Geometry check sheet. Reference: the model listing, model coordinates, mm. Round coordinates to 2 decimals unless told otherwise and drop trailing zeros. Order: outer loops, then holes, each group sorted by start corner. A loop starts at its lowest first (then second) coordinate and runs counter-clockwise, first axis right, second up. Notation, with made-up numbers: M 10.5,80 L 26.5,80 A17 ccw 26.5,100 Z; hole C 53,-10 d5. An arc over 180 degrees is marked long. Return JSON: item names as keys, results as strings. Group by question number.
Autodesk Inventor part; units mm, degrees
ref_plane "YZ Plane" through (0, 0, 0) normal (1, 0, 0) x (0, 1, 0)
ref_plane "XZ Plane" through (0, 0, 0) normal (0, 1, 0) x (-1, 0, 0)
ref_plane "XY Plane" through (0, 0, 0) normal (0, 0, 1) x (1, 0, 0)
sketch "Sketch1" plane through (0, 0, 0) normal (0, 1, 0) x (-1, 0, 0)
  line L0 (0, 0) -> (127, 0)
  line L1 (127, 0) -> (127, -152.4)
  line L2 (127, -152.4) -> (0, -152.4)
  line L3 (0, -152.4) -> (0, 0)
  line L4 (127, -65.405) -> (25.4, -65.405)
  line L5 (25.4, -65.405) -> (25.4, -86.995)
  line L6 (25.4, -86.995) -> (127, -86.995)
  line L7 (127, -86.995) -> (127, -65.405)
  dimension "d0" = 152.4
  dimension "d1" = 127
  dimension "d2" = 21.59
  dimension "d3" = 65.405
  dimension "d4" = 101.6
extrude "Extrusion1" add sketch "Sketch1" along normal blind 1.8542 contours L0 L1 L4 L5 L6 L2 L3
equation "\"d3\" = -0.5 * d2 + 0.5 * d0"
properties part number "paddle collection ramp"
Q1. Section check B-B on y = 1.1. Record the cut outline in (x, z) (3 decimals), plus the area to 3 significant figures.
Q2. Material ranges on line 1 along Z through (x, y) = (-106, 0.4) (3 decimals); line 2 along X through (y, z) = (1.7, -74), recorded low to high.
Q3. Section check C-C on z = -80. Record the cut outline in (x, y).
Q4. Section check A-A on x = -94. Record the cut outline in (y, z) (3 decimals), plus the area to 3 significant figures.
Geometry check:
{
 "1": {"outline": "M -127,-152.4 L 0,-152.4 L 0,0 L -127,0 L -127,-65.405 L -25.4,-65.405 L -25.4,-86.995 L -127,-86.995 Z", "area": "17,200 mm^2"},
 "2": {"line 1": "z = -152.4 to -86.995, -65.405 to 0", "line 2": "x = -25.4 to 0"},
 "3": {"outline": "M -25.4,0 L 0,0 L 0,1.85 L -25.4,1.85 Z"},
 "4": {"outline": "M 0,-152.4 L 1.854,-152.4 L 1.854,-86.995 L 0,-86.995 Z; M 0,-65.405 L 1.854,-65.405 L 1.854,0 L 0,0 Z", "area": "243 mm^2"}
}
